Print and shaded views of the part. All mm, measured from the part's lowest x, y and z. A direction names the side the tool comes from. Round coordinates to 2 decimals unless told otherwise and drop trailing zeros. Loops run counter-clockwise (first coordinate to the right, second up) from the corner with the lowest first, then second, coordinate; pieces in that order, holes last. Notation, with made-up numbers: (43, -31.75) - (92, -31.75) arc R20 ccw to (92, -23.75) - close; hole circle Ø2 at (-16, 29). An arc over 180 degrees is marked (long way). Answer as a JSON object with one key per item and string values.
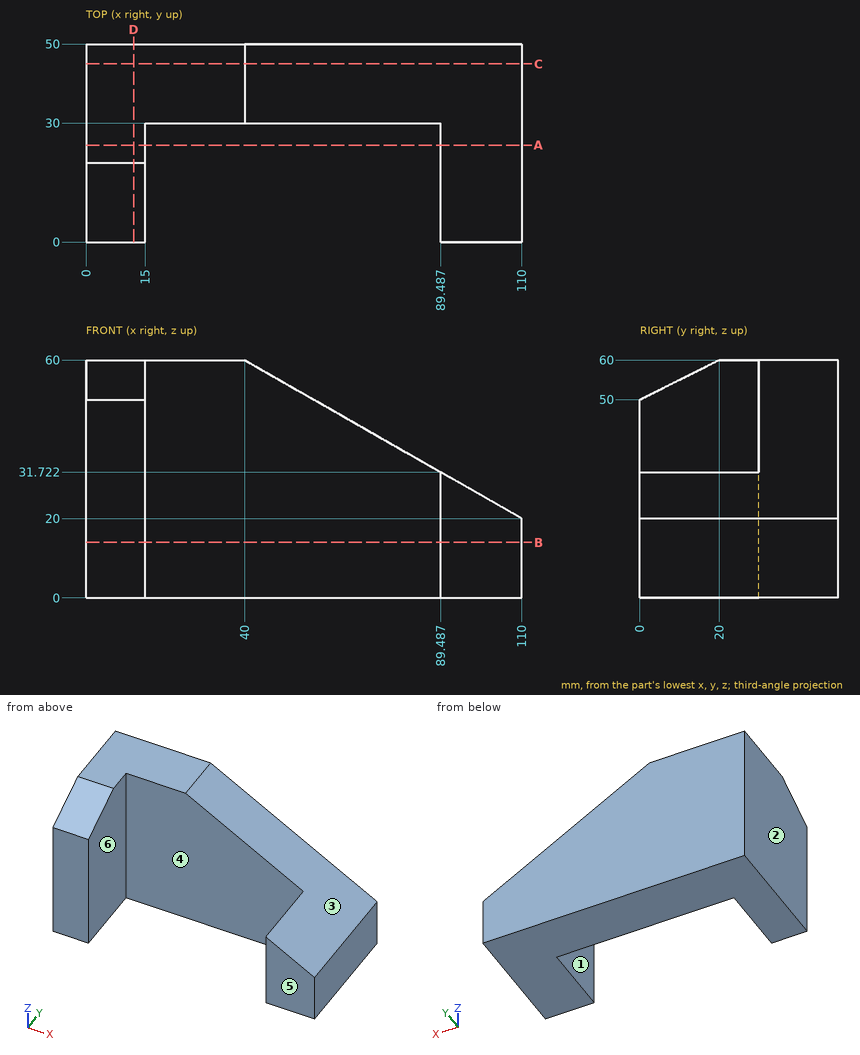
1) Probe probe 1 along X at (y, z) = (29, 9.5); probe 2 along Y at (x, z) = (80, 31); probe 3 along X at (y, z) = (6, 34). List the from-to ranges inside material, lowest first.
Values follow:
{"probe 1": "0 to 15, 89.49 to 110", "probe 2": "30 to 50", "probe 3": "0 to 15"}
2) Slice it at B-B on z = 14. List the corners of the cut face in (x, y), then the cut area to 3 significant figures.
Values follow:
{"outline": "(0, 0) - (15, 0) - (15, 30) - (89.49, 30) - (89.49, 0) - (110, 0) - (110, 50) - (0, 50) - close", "area": "3,270 mm²"}
3) Two-plate mould, pull along X, no slides. Class the marked faces 3, 4, 5 and 6: pulls with the +X half, pulls with the -X half, needs draft (parallel to the pull), parting line crosses it, or undercut.
Values follow:
{"face 3": "pulls with the +X half", "face 4": "undercut", "face 5": "needs draft", "face 6": "undercut"}
4) Slice it at A-A on y = 24.5. List the corners of the cut face in (x, z).
Values follow:
{"outline": "(0, 0) - (15, 0) - (15, 60) - (0, 60) - close; (89.49, 0) - (110, 0) - (110, 20) - (89.49, 31.72) - close"}
5) Slice it at C-C on y = 45. List the corners of the cut face in (x, z).
Values follow:
{"outline": "(0, 0) - (110, 0) - (110, 20) - (40, 60) - (0, 60) - close"}
6) Tool access for the marked faces 1 and 2: list every direction of +Z, -Z, +X, -X, +Y, -Y with a clear straight run to the whole face (end or side of a thin tool).
Values follow:
{"face 1": "+Z, -Z, -Y", "face 2": "+Z, -Z, -X, +Y, -Y"}
7) Drop flat-ended pins along their axis: P1, Ø8, axis at x = 39.5, z = 15, coming from the -Y side; P2, Ø3, axis at y = 17.5, z = 50, coming from the +X side; P3, Ø15, axis at y = 17, z = 31.5, coming from the +X side. Give the stop position or say it passes through.
Values follow:
{"P1": "y = 30", "P2": "x = 15", "P3": "x = 103"}
8) Slice it at D-D on x = 12. List the corners of the cut face in (y, z), then the cut area to 3 significant figures.
Values follow:
{"outline": "(0, 0) - (50, 0) - (50, 60) - (20, 60) - (0, 50) - close", "area": "2,900 mm²"}
